Build history of the part. All positions in model axes, mm. Coordinates: 2 decimals unless noted, no trailing zeros. Order: outer loops, then holes, each group sorted by start corner. A loop starts at its lowest first (then second) coordinate and runs counter-clockwise, first axis right, second up. Notation, with made-up numbers: (19, 54) - (69, 54) arc R32 cw to (69, 90) - close; hole circle Ø2 at (55, 67.5). An arc over 180 degrees is marked (long way). Return JSON: item names as keys, results as strings.
from build123d import *

# Parameters (mm, degrees)
F0_W     = 65.532
F0_H     = 123.952
F1_DEPTH = 38.227
F3_D     = 5.1054


with BuildPart() as f1:
    # F0 (on Front) → F1 (new body)
    with BuildSketch(Plane.XZ):
        Rectangle(F0_W, F0_H)
    extrude(amount=-F1_DEPTH)

    # F3 (through all)
    with Locations(Plane.XZ):
        with Locations((0, 23.8125), (0, -23.8125)):
            Hole(F3_D / 2)


solid = f1.part
1. Mould opens along Z. For faces 1 (the flat face through (32.766, 19, -1)), 2 (the flat face through (0, 19, 61.976)), 3 (the cylindrical face through (-1.37, 19.38, -21.66)), 4 (the cylindrical face through (-1.372, 19.381, 25.965)) say: pulls with the +Z half, pulls with the -Z half, needs draft (parallel to the pull), parting line crosses it, or undercut.
Check values:
{"face 1": "needs draft", "face 2": "pulls with the +Z half", "face 3": "undercut", "face 4": "undercut"}
2. Cut at A-A on x = 0. Give the cut face in (y, z).
Check values:
{"outline": "(0, -61.98) - (38.23, -61.98) - (38.23, -26.37) - (0, -26.37) - close; (0, -21.26) - (38.23, -21.26) - (38.23, 21.26) - (0, 21.26) - close; (0, 26.37) - (38.23, 26.37) - (38.23, 61.98) - (0, 61.98) - close"}
3. Probe L1, parallel to Z at x = 0, y = 30; L2, parallel to Z at x = -1, y = 17.5; L3, parallel to X at y = 36.5, z = -22. List the from-to ranges inside material, lowest first.
Check values:
{"L1": "-61.98 to -26.37, -21.26 to 21.26, 26.37 to 61.98", "L2": "-61.98 to -26.16, -21.46 to 21.46, 26.16 to 61.98", "L3": "-32.77 to -1.8, 1.8 to 32.77"}
